Source: three-view drawing plus pictorial views. Frame: mm from the lowest corner of the part. Coordinates: 2 decimals unless noted, no trailing zeros. Write each loop counter-clockwise with the first axis right and the second up, starting at its lowest first coordinate (ties: lowest second). Pieces come first, ordered by that corner, then holes. Notation, with made-up numbers: (23.5, 70.5) - (39.5, 70.5) arc R13 cw to (39.5, 77.5) - close; hole circle Ø2 at (-23.75, 65.25). An arc over 180 degrees is marked (long way). Put each result on its own line as item: value.
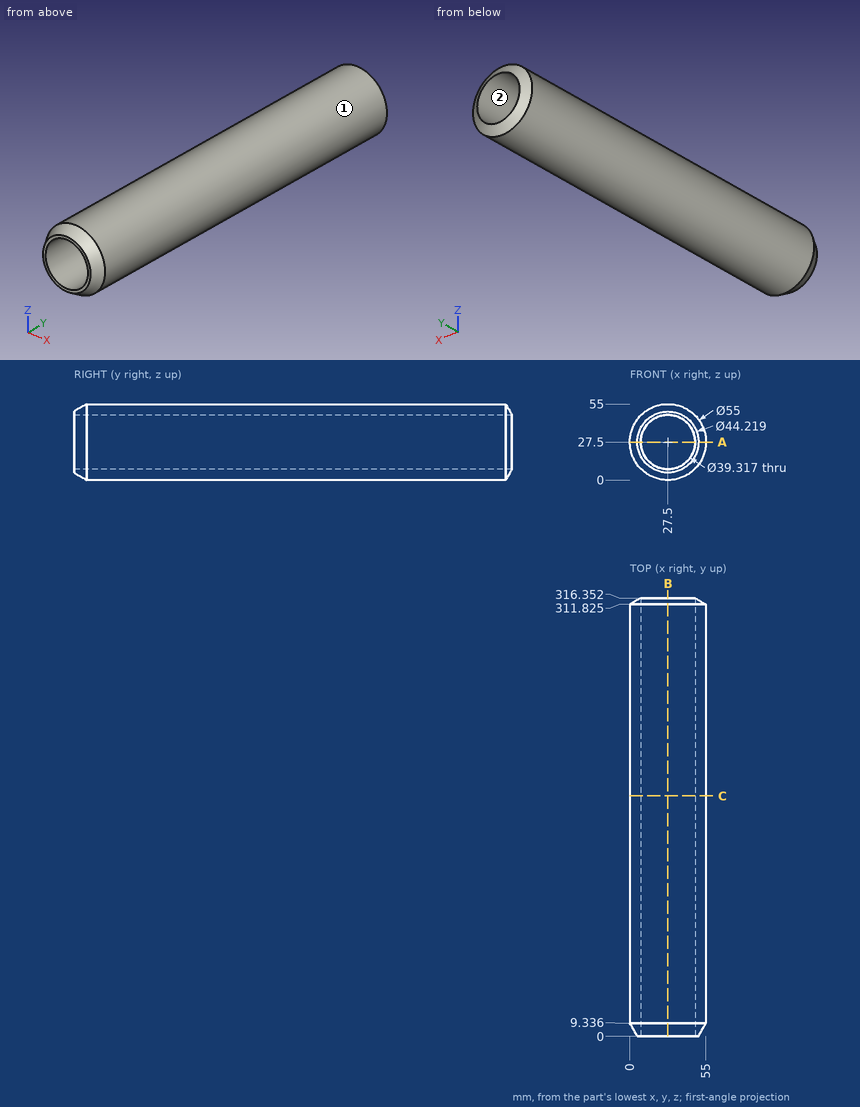
1. Section query B-B (x = 27.5). Return loops of the section in (y, z) (1 decimal).
Answer below:
outline: (0, 5.4) - (9.3, 0) - (311.8, 0) - (316.4, 7.8) - (0, 7.8) - close; (0, 47.2) - (316.4, 47.2) - (311.8, 55) - (9.3, 55) - (0, 49.6) - close
2. Section query A-A (z = 27.5). Return loops of the section in (x, y) (1 decimal).
Answer below:
outline: (0, 9.3) - (5.4, 0) - (7.8, 0) - (7.8, 316.4) - (0, 311.8) - close; (47.2, 0) - (49.6, 0) - (55, 9.3) - (55, 311.8) - (47.2, 316.4) - close
3. Pin query (flat end, axial travel): pin 1 Ø1 at (x, y) = (6, 231.5) entering from +Z (1 decimal); pin 2 Ø3 at (x, y) = (34, 153) entering from -Z; pin 3 Ø8 at (x, y) = (20.5, 226.5) entering from +Z. Return the tip coordinate at first contact, or that it passes through.
Answer below:
pin 1: stops at z = 45.3
pin 2: stops at z = 0.46
pin 3: stops at z = 54.84
4. Mould query, pull axis X, two halves, no side actions, for the marked faces 1 and 2. Classes: +X half, -X half, draft (parallel to the pull), parting line (faces both ways), or undercut.
Answer below:
face 1: parting line
face 2: undercut
5. Section query C-C (y = 173.5). Return loops of the section in (x, z).
Answer below:
outline: circle Ø55 at (27.5, 27.5); hole circle Ø39.32 at (27.5, 27.5)
6. Ray query, probe 1 along X at (y, z) = (109.5, 27.5); probe 2 along Z at (x, y) = (18, 28.5) (1 decimal); probe 3 along Z at (x, y) = (31, 127) (1 decimal). Return the intervals inside material, ascending. Write a range as from..to.
Answer below:
probe 1: x = 0..7.84, 47.16..55
probe 2: z = 1.7..10.3, 44.7..53.3
probe 3: z = 0.2..8.2, 46.8..54.8
